Verification items for the finished model (mm, model axes). A direction names the side the tool comes from. Round coordinates to 2 decimals unless told otherwise and drop trailing zeros. Write each loop counter-clockwise with the first axis right and the second up, starting at its lowest first coordinate (ties: lowest second). Pieces come first, ordered by that corner, then holes. Notation, with made-up numbers: (14, 15.25) - (39, 15.25) arc R16 ccw to (39, 37.25) - close; hole circle Ø3 at (35, 84). An arc over 180 degrees is marked (long way). Write each question's results on one line, items separated by ' | '.
```python
from build123d import *

# Parameters (mm, degrees)
F4_W      = 35
F4_H      = 18.6
F5_DEPTH  = 2
F4_W_2    = 2
F4_H_2    = 2
F6_DEPTH  = 37
F7_DEPTH  = 14.3
F8_W      = 2
F8_H      = 22.7
F9_DEPTH  = 12.3
F11_DEPTH = 22.6
F12_R     = 2
F14_DEPTH = 1
F15_SIZE  = 0.99999
F17_DEPTH = 1
F18_SIZE  = 0.99999


# Not quite as in the source:
# - a fillet or chamfer is up to 0.001 mm smaller than in the source, because OpenCascade refuses the exact size


with BuildPart() as f5:
    # F4 (on Top) → F5 (new body)
    with BuildSketch(Plane.XY):
        with Locations((17.5, -11.3)):
            Rectangle(F4_W, F4_H)
    extrude(amount=F5_DEPTH)

    # F4 (on Top) → F6 (join)
    with BuildSketch(Plane.XY):
        with Locations((36, -11.3)):
            Rectangle(F4_W_2, F4_H)
        with Locations((36, -21.6)):
            Rectangle(F4_W_2, F4_H_2)
        with Locations((36, -1)):
            Rectangle(F4_W_2, F4_H_2)
    extrude(amount=F6_DEPTH)

    # F4 (on Top) → F7 (join)
    with BuildSketch(Plane.XY):
        with Locations((17.5, -1)):
            Rectangle(F4_W, F4_H_2)
        with Locations((17.5, -21.6)):
            Rectangle(F4_W, F4_H_2)
    extrude(amount=F7_DEPTH)

    # F8 (on face) → F9 (join)
    with BuildSketch(Plane(origin=(35, 0, 0), x_dir=(0, -1, 0), z_dir=(-1, 0, 0))):
        with Locations((1, 25.65)):
            Rectangle(F8_W, F8_H)
        with Locations((21.6, 25.65)):
            Rectangle(F8_W, F8_H)
    extrude(amount=F9_DEPTH)

    # F10 (on face) → F11 (cut)
    with BuildSketch(Plane.XZ.offset(22.6)):
        Polygon((8.2561088494, 0), (0, 14.3), (0, 0), align=None)
        Polygon((37, 37), (22.7, 37), (37, 28.7438911506), align=None)
    extrude(amount=-F11_DEPTH, mode=Mode.SUBTRACT)

    # F12
    f12_edges = [f5.edges().sort_by_distance(p)[0] for p in [
        (37, -11.3, 0),
        (22.628054, -22.6, 0),
        (37, -22.6, 14.371946),
        (37, 0, 14.371946),
        (22.628054, 0, 0),
        (8.256109, -11.3, 0),
        (37, -11.3, 28.743891),
    ]]
    fillet(f12_edges, radius=F12_R)

    # F13 (on face) → F14 (join)
    with BuildSketch(Plane.XZ.offset(2)):
        Polygon((25.2, 35.556624327), (22.7, 37), (22.7, 27), (25.2, 27), align=None)
        Polygon((10, 11.8), (10, 14.3), (0, 14.3), (1.443375673, 11.8), align=None)
    extrude(amount=F14_DEPTH)

    # F15 (size 1 in the source; OpenCascade refuses exactly that, so slightly less here)
    f15_edges = [f5.edges().sort_by_distance(p)[0] for p in [
        (23.95, -3, 27),
        (5.721688, -3, 11.8),
        (22.7, -3, 32),
        (5, -3, 14.3),
    ]]
    chamfer(f15_edges, length=F15_SIZE)

    # F16 (on face) → F17 (join)
    with BuildSketch(Plane(origin=(0, -20.6, 0), x_dir=(-1, 0, 0), z_dir=(0, 1, 0))):
        Polygon((-22.7, 27), (-22.7, 37), (-25.2, 35.556624327), (-25.2, 27), align=None)
        Polygon((0, 14.3), (-10, 14.3), (-10, 11.8), (-1.443375673, 11.8), align=None)
    extrude(amount=F17_DEPTH)

    # F18 (size 1 in the source; OpenCascade refuses exactly that, so slightly less here)
    f18_edges = [f5.edges().sort_by_distance(p)[0] for p in [
        (5.721688, -19.6, 11.8),
        (5, -19.6, 14.3),
        (22.7, -19.6, 32),
        (23.95, -19.6, 27),
    ]]
    chamfer(f18_edges, length=F18_SIZE)


solid = f5.part
```
(1) Thickness scan on L1, parallel to Y at x = 19.5, z = 12; L2, parallel to Z at x = 15, y = -13; L3, parallel to X at y = -16.75, z = 3. Record the ranges inside material, lowest first.
Answer:
L1: -22.6 to -20.6, -2 to 0 | L2: 0 to 2 | L3: 35 to 37
(2) Section check C-C (y = -14.75). Record the cut outline in (x, z).
Answer:
outline: (7.1, 2) - (7.68, 1) arc R2 ccw to (9.41, 0) - (35, 0) arc R2 ccw to (37, 2) - (37, 27.59) arc R2 ccw to (36, 29.32) - (35, 29.9) - (35, 2) - close
(3) Section check A-A (z = 33.5). Record the cut outline in (x, y), plus the area to 3 significant figures.
Answer:
outline: (22.7, -22.6) - (28.76, -22.6) - (28.76, -20.6) - (25.2, -20.6) - (25.2, -19.6) - (23.7, -19.6) - (22.7, -20.6) - close; (22.7, -2) - (23.7, -3) - (25.2, -3) - (25.2, -2) - (28.76, -2) - (28.76, 0) - (22.7, 0) - close | area: 28.2 mm2
(4) Set-up check for faces 4 (the flat face through (25.2, -2.5, 31.2)), 5 (the flat face through (24.2, -2.5, 27.5)), 6 (the cylindrical face through (8.398, -11.146, 0.275)), 7 (the flat face through (5.1, -2.5, 13.8)), 8 (the flat face through (22, 0, 11)): record each of +Z, -Z, +X, -X, +Y, -Y from which the full face is reachable in a straight line by a thin tool's end or side.
Answer:
face 4: +Z | face 5: -X | face 6: -Z, -X, +Y, -Y | face 7: +Z, -X | face 8: +Z, -Z, +X, -X, +Y
(5) Section check D-D (z = 26.5). Record the cut outline in (x, y).
Answer:
outline: (22.7, -22.6) - (35, -22.6) arc R2 ccw to (37, -20.6) - (37, -2) arc R2 ccw to (35, 0) - (22.7, 0) - (22.7, -2) - (35, -2) - (35, -20.6) - (22.7, -20.6) - close
(6) Go/stop test with flat-tipped pins: pin 1 Ø3 at (y, z) = (-3, 25) entering from -X; pin 2 Ø5 at (x, y) = (19.5, -14) entering from +Z; pin 3 Ø0.6 at (x, y) = (6, -21) entering from +Z; pin 4 Ø12 at (y, z) = (-7, 28.5) entering from +X. Record where each tip stops, or that it passes through.
Answer:
pin 1: x = 22.7 | pin 2: z = 2 | pin 3: z = 14.3 | pin 4: x = 37
(7) Mould release check, pull along Y, two halves, no side actions. Record for faces 1 (the flat face through (22.7, -1, 26)), 2 (the cylindrical face through (36.43, -22, 16.14)), 3 (the flat face through (5.4, -2.5, 12.3)): released by +Y, released by -Y, zero draft, split by the parting line, or undercut.
Answer:
face 1: zero draft | face 2: released by -Y | face 3: undercut
